Check sheet for the modelled part. Datum: model origin and axes. Units: mm. A direction names the side the tool comes from. Give positions to 0.01 mm unless a question says otherwise; leave off trailing zeros. Write each loop counter-clockwise with the first axis right and the second up, starting at its lowest first coordinate (ties: lowest second). Pieces come first, ordered by that corner, then holes. Notation, with made-up numbers: M -9,46.5 L 20,46.5 A25 cw 20,75.5 Z; hole C 53.25,-35 d3. An arc over 180 degrees is marked long. Write item = value, one per line. Start each with the question number.
1) Sectioned sample at D-D, the plane y = -4. Record the cut outline in (x, z) (3 decimals), then the cut area to 3 significant figures.
2) Draft check along Y on faces 4 (the face through (0.07, 3.174, -2.63)), 5 (the face through (-1.077, 25.477, -2.63)), 6 (the face through (-5, 0, 0)), 7 (the face through (0.162, 7.233, -2.63)). Enter one of: pulls with the +Y half, pulls with the -Y half, needs draft (parallel to the pull), parting line crosses it, or undercut.
3) Set-up check for faces 1 (the face through (7.366, -10, -3)), 2 (the face through (-3.175, -12, -3)), 3 (the face through (-5, 0, -5.334)): record each of +Z, -Z, +X, -X, +Y, -Y from which the full face is reachable in a straight line by a thin tool's end or side.
4) Sectioned sample at A-A, the plane z = -3.75. Record the cut outline in (x, y) (3 decimals).
5) Scan lines: L1, parallel to X at y = -14, z = -4 (3 decimals); L2, parallel to X at y = 3.5, z = -2.3; L3, parallel to X at y = 6, z = -2.4. Record each from-to range of solid material in increasing order.
6) Sectioned sample at C-C, the plane y = 18.5. Record the cut outline in (x, z).
7) Gauge pin test, flat ends, axial feed: pin 1 (1.6 mm diameter, centred on y = -11.5, z = -1.5, fed in from +X); pin 2 (3 mm diameter, centred on y = -5.5, z = -4.5, fed in from -X); pin 3 (1.6 mm diameter, centred on y = -12.5, z = -2, fed in from -X). Record the tip position at first contact, or that the pin passes through.
8) Sectioned sample at B-B, the plane x = 0. Record the cut outline in (y, z) (3 decimals), then the cut area to 3 significant figures.
from build123d import *

# Parameters (mm, degrees)
BOSS_EXTRUDE1_DEPTH = 5.334
CUT_EXTRUDE1_DEPTH  = 37.454787834


with BuildPart() as part:
    # Sketch1 → Boss-Extrude1 (new body)
    with BuildSketch(Plane.XY):
        with BuildLine():
            Line((-3.175, 0), (-3.175, -25.301568627))
            ThreePointArc((-3.175, -25.301568627), (0, 25.5), (3.175, -25.301568627))
            Line((3.175, -25.301568627), (3.175, 0))
            ThreePointArc((3.175, 0), (0, 3.175), (-3.175, 0))
        make_face()
    extrude(amount=-BOSS_EXTRUDE1_DEPTH)

    # Sketch3 → Cut-Extrude1 (cut, through all)
    with BuildSketch(Plane.XY):
        with BuildLine():
            Line((-7.365810735, -0.130956725), (-7.365810735, -19.019753779))
            ThreePointArc((-7.365810735, -19.019753779), (0, 20.143209644), (7.365810735, -19.019753779))
            Line((7.365810735, -19.019753779), (7.365810735, -0.130956725))
            ThreePointArc((7.365810735, -0.130956725), (0, 7.23485401), (-7.365810735, -0.130956725))
        make_face()
    extrude(amount=-CUT_EXTRUDE1_DEPTH, mode=Mode.SUBTRACT)


solid = part.part
Data:
q1.outline = M -25.184,-5.334 L -19.902,-5.334 L -19.902,0 L -25.184,0 Z; M -7.366,-5.334 L -3.175,-5.334 L -3.175,0 L -7.366,0 Z; M 3.175,-5.334 L 7.366,-5.334 L 7.366,0 L 3.175,0 Z; M 19.902,-5.334 L 25.184,-5.334 L 25.184,0 L 19.902,0 Z
q1.area = 101 mm2
q2.face_4 = pulls with the -Y half
q2.face_5 = parting line crosses it
q2.face_6 = needs draft
q2.face_7 = undercut
q3.face_1 = +Z, -Z
q3.face_2 = +Z, -Z, -Y
q3.face_3 = -Z, +X, -X, +Y, -Y
q4.outline = M -3.175,-25.302 L -3.175,0 A3.175 cw 3.175,0 L 3.175,-25.302 A25.5 ccw long Z; hole M -7.366,-19.02 L -7.366,-0.131 A7.366 cw 7.366,-0.131 L 7.366,-19.02 A20.274 ccw long Z
q5.L1 = -21.313 to -14.788, -7.366 to -3.175, 3.175 to 7.366, 14.788 to 21.313
q5.L2 = -25.26 to -19.95, -6.41 to 6.41, 19.95 to 25.26
q5.L3 = -24.78 to -19.32, -4.08 to 4.08, 19.32 to 24.78
q6.outline = M -17.55,-5.33 L -8,-5.33 L -8,0 L -17.55,0 Z; M 8,-5.33 L 17.55,-5.33 L 17.55,0 L 8,0 Z
q7.pin_1 = 23.15
q7.pin_2 = -25.18
q7.pin_3 = -22.66
q8.outline = M 3.175,-5.334 L 7.235,-5.334 L 7.235,0 L 3.175,0 Z; M 20.143,-5.334 L 25.5,-5.334 L 25.5,0 L 20.143,0 Z
q8.area = 50.2 mm2
